from build123d import *

# Parameters (mm, degrees)
SKETCH1_R                = 5.5
BOSS_EXTRUDE1_DEPTH      = 10
SKETCH1_3_R              = 5.5
SKETCH1_3_R_2            = 2.5
BOSS_EXTRUDE2_DEPTH      = 2
SKETCH1_4_R              = 2.5
BOSS_EXTRUDE3_DEPTH      = 5
BOSS_EXTRUDE4_DEPTH      = 5
SKETCH4_W                = 20
SKETCH4_H                = 80
BOSS_EXTRUDE5_DEPTH      = 20
SKETCH5_W                = 20
SKETCH5_H                = 2
BOSS_EXTRUDE6_DEPTH      = 10
BOSS_EXTRUDE6_DEPTH_BACK = 30
SKETCH7_W                = 5
SKETCH7_H                = 10
CUT_EXTRUDE1_DEPTH       = 78
FILLET1_R                = 10
SKETCH9_R                = 2.5
CUT_EXTRUDE2_DEPTH       = 38.5
SKETCH14_R               = 1.5
BOSS_EXTRUDE8_DEPTH      = 3


with BuildPart() as part:
    # Sketch1 → Boss-Extrude1 (new body)
    with BuildSketch(Plane.XY):
        with BuildLine():
            Line((31.5, 0), (31.5, 40))
            Line((31.5, 40), (-31.5, 40))
            Line((-31.5, 40), (-31.5, 0))
            ThreePointArc((-31.5, 0), (0, -31.5), (31.5, 0))
        make_face()
        with Locations((17.67766953, -17.67766953)):
            Circle(SKETCH1_R, mode=Mode.SUBTRACT)
        with Locations((-17.67766953, -17.67766953)):
            Circle(SKETCH1_R, mode=Mode.SUBTRACT)
        with Locations((-17.67766953, 17.67766953)):
            Circle(SKETCH1_R, mode=Mode.SUBTRACT)
        with Locations((17.67766953, 17.67766953)):
            Circle(SKETCH1_R, mode=Mode.SUBTRACT)
    extrude(amount=BOSS_EXTRUDE1_DEPTH)

    # Sketch1_3 → Boss-Extrude2 (add)
    with BuildSketch(Plane.XY):
        with Locations((17.67766953, 17.67766953)):
            Circle(SKETCH1_3_R)
        with Locations((17.67766953, 17.67766953)):
            Circle(SKETCH1_3_R_2, mode=Mode.SUBTRACT)
        with Locations((17.67766953, -17.67766953)):
            Circle(SKETCH1_3_R)
        with Locations((17.67766953, -17.67766953)):
            Circle(SKETCH1_3_R_2, mode=Mode.SUBTRACT)
        with Locations((-17.67766953, -17.67766953)):
            Circle(SKETCH1_3_R)
        with Locations((-17.67766953, -17.67766953)):
            Circle(SKETCH1_3_R_2, mode=Mode.SUBTRACT)
        with Locations((-17.67766953, 17.67766953)):
            Circle(SKETCH1_3_R)
        with Locations((-17.67766953, 17.67766953)):
            Circle(SKETCH1_3_R_2, mode=Mode.SUBTRACT)
    extrude(amount=BOSS_EXTRUDE2_DEPTH)

    # Sketch1_4 → Boss-Extrude3 (add)
    with BuildSketch(Plane.XY):
        with Locations((0, 25)):
            Circle(SKETCH1_4_R)
    extrude(amount=-BOSS_EXTRUDE3_DEPTH)

    # Sketch2 → Boss-Extrude4 (add)
    with BuildSketch(Plane(origin=(0, 40, 0), x_dir=(1, 0, 0), z_dir=(0, 1, 0))):
        Polygon((-32.5, -10), (31.5, -10), (32.5, -10), (32.5, 15), (-32.5, 15), align=None)
    extrude(amount=-BOSS_EXTRUDE4_DEPTH)

    # Sketch4 → Boss-Extrude5 (add)
    with BuildSketch(Plane.XY.offset(10)):
        Rectangle(SKETCH4_W, SKETCH4_H)
    extrude(amount=BOSS_EXTRUDE5_DEPTH)

    # Sketch5 → Boss-Extrude6 (add, two sides)
    with BuildSketch(Plane(origin=(10, 0, 0), x_dir=(0, 0, -1), z_dir=(1, 0, 0))) as boss_extrude6_sk:
        with Locations((-20, -39)):
            Rectangle(SKETCH5_W, SKETCH5_H)
    extrude(amount=BOSS_EXTRUDE6_DEPTH)
    extrude(boss_extrude6_sk.sketch, amount=-BOSS_EXTRUDE6_DEPTH_BACK)

    # Sketch7 → Cut-Extrude1 (cut)
    with BuildSketch(Plane(origin=(0, 40, 0), x_dir=(1, 0, 0), z_dir=(0, 1, 0))):
        with Locations((-7.5, -20)):
            Rectangle(SKETCH7_W, SKETCH7_H)
        with Locations((7.5, -20)):
            Rectangle(SKETCH7_W, SKETCH7_H)
    extrude(amount=-CUT_EXTRUDE1_DEPTH, mode=Mode.SUBTRACT)

    # Fillet1
    fillet1_edges = [part.edges().sort_by_distance(p)[0] for p in [
        (-20, -39, 30),
        (20, -39, 30),
    ]]
    fillet(fillet1_edges, radius=FILLET1_R)

    # Sketch9 → Cut-Extrude2 (cut, through all)
    with BuildSketch(Plane(origin=(5, 0, 0), x_dir=(0, 0, -1), z_dir=(1, 0, 0))):
        with Locations((-20, 12.5)):
            Circle(SKETCH9_R)
    extrude(amount=-CUT_EXTRUDE2_DEPTH, mode=Mode.SUBTRACT)

    # Sketch14 → Boss-Extrude8 (add)
    with BuildSketch(Plane(origin=(0, 0, -15), x_dir=(-1, 0, 0), z_dir=(0, 0, -1))):
        with BuildLine():
            Line((32.5, 62), (-32.5, 62))
            ThreePointArc((-32.5, 62), (-43.5, 51), (-32.5, 40))
            Line((-32.5, 40), (32.5, 40))
            ThreePointArc((32.5, 40), (43.5, 51), (32.5, 62))
        make_face()
        with Locations((-22, 51)):
            Circle(SKETCH14_R, mode=Mode.SUBTRACT)
        with Locations((22, 51)):
            Circle(SKETCH14_R, mode=Mode.SUBTRACT)
    extrude(amount=-BOSS_EXTRUDE8_DEPTH)


solid = part.part
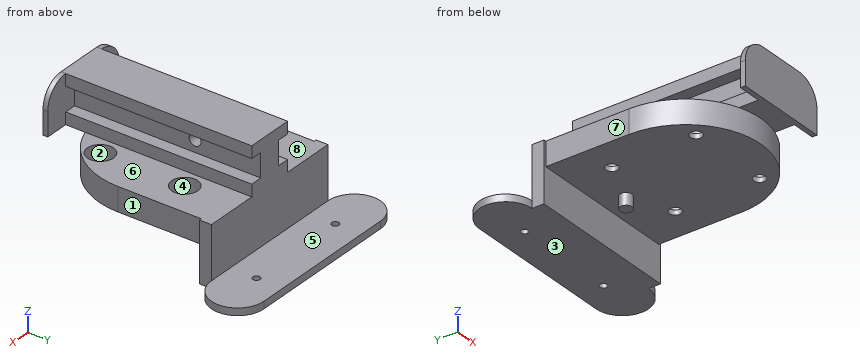
Check sheet for the modelled part. Datum: model origin and axes. Units: mm. Face numbers are marked on the shaded views. A direction names the side the tool comes from. Round coordinates to 2 decimals unless told otherwise and drop trailing zeros. Loops run counter-clockwise (first coordinate to the right, second up) from the corner with the lowest first, then second, coordinate; pieces in that order, holes last. Notation, with made-up numbers: (-16.75, 20.5) -> (8.25, 20.5) arc R20 ccw to (8.25, 36.5) -> close; hole circle Ø8 at (58.5, 77.5). An arc over 180 degrees is marked (long way). Put each result on its own line as item: value. Start each with the question number.
1. Section check A-A (y = 51). Enter the section's corners in (x, z).
2. Gauge pin test, flat ends, axial feed: pin 1 (5 mm diameter, centred on x = 25.5, y = 25, fed in from -Z); pin 2 (1.6 mm diameter, centred on y = -39, z = 13.5, fed in from -X); pin 3 (8 mm diameter, centred on y = 24, z = 6, fed in from +X). Record the tip position at first contact, or that the pin passes through.
3. Section check D-D (z = 7.5). Enter the section's corners in (x, y), plus the area to 3 significant figures.
4. Section check C-C (x = -14). Enter the section's corners in (y, z).
5. Access from +Z, -Z, +X, -X, +Y, -Y to the whole of each face (thin tool, end or side, straight path). Record for the marked faces 5, 6, 7 and 8.
6. Section check B-B (z = -3). Enter the section's corners in (x, y).
7. Draft check along X on the marked faces 1, 2, 3 and 4. Enter one of: +X half, -X half, draft (parallel to the pull), parting line (faces both ways), or undercut.
8. Scan lines: probe 1 along Y at (x, z) = (-22, -13); probe 2 along X at (y, z) = (26, 16); probe 3 along Z at (x, y) = (29, 37). Record each from-to range of solid material in increasing order.
Findings:
1. outline: (-43.5, -15) -> (-23.5, -15) -> (-23.5, -12) -> (-43.5, -12) -> close; (-20.5, -15) -> (20.5, -15) -> (20.5, -12) -> (-20.5, -12) -> close; (23.5, -15) -> (43.5, -15) -> (43.5, -12) -> (23.5, -12) -> close
2. pin 1: stops at z = 0
2. pin 2: stops at x = -20
2. pin 3: stops at x = 31.5
3. outline: (-32.5, 35) -> (-31.5, 35) -> (-31.5, 0) arc R31.5 ccw to (31.5, 0) -> (31.5, 35) -> (32.5, 35) -> (32.5, 40) -> (-32.5, 40) -> close; hole circle Ø11 at (-17.68, -17.68); hole circle Ø11 at (-17.68, 17.68); hole circle Ø11 at (17.68, -17.68); hole circle Ø11 at (17.68, 17.68)
3. area: 3,710 mm^2
4. outline: (-40, 10) -> (-38, 10) -> (-38, 29.17) -> (-40, 29.17) -> close; (-28.22, 0) -> (35, 0) -> (35, -15) -> (62, -15) -> (62, -12) -> (40, -12) -> (40, 10) -> (21.77, 10) -> (21.77, 2) -> (13.59, 2) -> (13.59, 10) -> (-13.59, 10) -> (-13.59, 2) -> (-21.77, 2) -> (-21.77, 10) -> (-28.22, 10) -> close
5. face 5: +Z, +X, -X, +Y
5. face 6: +Z, +X, +Y
5. face 7: +Z, -Z, -X, -Y
5. face 8: +Z, -X, +Y
6. outline: (-32.5, 35) -> (32.5, 35) -> (32.5, 40) -> (-32.5, 40) -> close; circle Ø5 at (0, 25)
7. face 1: +X half
7. face 2: undercut
7. face 3: draft
7. face 4: undercut
8. probe 1: y = 35 to 49.5, 52.5 to 62
8. probe 2: x = -5 to 5
8. probe 3: z = -15 to 10
